The listing builds one solid part. Answer for the finished solid, in the listing's coordinates (mm). A direction names the side the tool comes from. Round coordinates to 2 decimals unless told otherwise and drop trailing zeros. Write each loop counter-clockwise with the first axis right and the second up, starting at its lowest first coordinate (ties: lowest second). Pieces come first, ordered by that corner, then holes.
Item 1: Find section C-C on z = 15. Give the vertices of the cut face in (x, y) (1 decimal).
Item 2: Find section B-B on y = 9. Give the vertices of the cut face in (x, z), then the cut area to 3 significant figures.
Item 3: A tool of negligible diameter and unlimited length cuts with its end or side. For faces 1 (the face through (13.694, 27.716, 14.79)), 2 (the face through (8.58, 15.86, 14.79)), 3 (the face through (14.315, 18.679, 14.79)), from which of +Z, -Z, +X, -X, +Y, -Y can it reach the whole face along a straight path? Write none if from no direction.
Item 4: Each of these flat-tipped pins is pushed along its axis until it touches: pin 1 (5 mm diameter, centred on y = 19, z = 20.5, fed in from -X); pin 2 (8 mm diameter, centred on x = 22.5, z = 10, fed in from +Y); pin 3 (5 mm diameter, centred on y = 25.5, z = 26.5, fed in from +X). Where does it stop, or does it pass through?
Item 5: For a pull along Y with two mould halves and no side action, classify faces 4 (the face through (17, 0, 15)), 5 (the face through (7.846, 28.994, 14.79)), 6 (the face through (4.78, 3.05, 14.79)) as +Y half, -Y half, draft (parallel to the pull), parting line (faces both ways), or undercut.
Item 6: Find section A-A on x = 7.5. Give the vertices of the cut face in (y, z).
Item 7: Find the intervals of material crossed by probe 1 along Y at (x, z) = (27.25, 19.5); probe 2 along X at (y, z) = (4.25, 15); probe 3 along X at (y, z) = (16.5, 23.25), in increasing order.
Item 8: Find section D-D on z = 26.5. Give the vertices of the cut face in (x, y) (1 decimal), then the cut area to 3 significant figures.
Autodesk Inventor part; units mm, degrees
ref_plane "YZ Plane" through (0, 0, 0) normal (1, 0, 0) x (0, 1, 0)
ref_plane "XZ Plane" through (0, 0, 0) normal (0, 1, 0) x (-1, 0, 0)
ref_plane "XY Plane" through (0, 0, 0) normal (0, 0, 1) x (1, 0, 0)
sketch "Szkic1" plane through (0, 0, 0) normal (0, 0, 1) x (1, 0, 0)
  line L0 (0, -6.7527) -> (0, 35.3194)
  line L1 (0.8414, 3.8525) -> (6.4011, 29.3091)
  line L2 (6.4011, 29.3091) -> (9.3321, 28.669)
  line L3 (9.3321, 28.669) -> (3.9978, 4.2447)
  line L4 (5.9517, 3.818) -> (11.286, 28.2423)
  line L5 (11.286, 28.2423) -> (16.1709, 27.1754)
  arc A0 (3.9978, 4.2447) -> (5.9517, 3.818) centre (4.9747, 4.0314) ccw
  line L6 (16.1709, 27.1754) -> (12.4071, 9.942)
  line L7 (13.9707, 8) -> (30.48, 8)
  arc A1 (12.4071, 9.942) -> (13.9707, 8) centre (13.9707, 9.6005) ccw
  line L8 (3.9433, 0) -> (30.48, 0)
  line L9 (30.48, 0) -> (30.48, 8)
  arc A2 (0.8414, 3.8525) -> (3.9433, 0) centre (3.9433, 3.175) ccw
  point P0 (0, 0)
  dimension "d0" = 12.32
  dimension "d1" = 3
  dimension "d2" = 30
  dimension "d3" = 5
  dimension "d4" = 8
  dimension "d5" = 25
  dimension "d6" = 2
  dimension "d7" = 30.48
  dimension "d8" = 1.6005
  dimension "d9" = 3.175
extrude "Wyciągnięcie proste1" add sketch "Szkic1" along normal blind 30
sketch "Szkic2" plane through (13.9707, 8, 0) normal (0, 1, 0) x (1, 0, 0)
  circle A0 centre (8.4108, -15) radius 2.25
  point P0 (-13.9707, 0)
  dimension "d12" = 4.5
extrude "Wyciągnięcie proste2" cut sketch "Szkic2" against normal blind 30
sketch "Szkic3" plane through (16.1709, 27.1754, 30) normal (0.9769712, -0.2133714, 0) x (0, 0, -1)
  circle A0 centre (15, -6.4184) radius 1.45
  point P0 (30, -30)
  dimension "d15" = 2.9
extrude "Wyciągnięcie proste3" cut sketch "Szkic3" against normal up to next
properties part number "lustereczko"
Check values:
1. outline: (0.8, 3.9) arc R3.2 ccw to (3.9, 0) - (20.1, 0) - (20.1, 8) - (14, 8) arc R1.6 cw to (12.4, 9.9) - (14.5, 19.5) - (9.6, 20.6) - (6, 3.8) arc R1 cw to (4, 4.2) - (9.3, 28.7) - (6.4, 29.3) - close; (10.2, 23.4) - (15.1, 22.3) - (16.2, 27.2) - (11.3, 28.2) - close; (24.6, 0) - (30.5, 0) - (30.5, 8) - (24.6, 8) - close
2. outline: (1.97, 0) - (5.04, 0) - (5.04, 30) - (1.97, 30) - close; (7.08, 0) - (12.49, 0) - (12.49, 30) - (7.08, 30) - close
2. area: 254 mm2
3. face 1: +Z, -Z, +X, +Y
3. face 2: +Z, -Z
3. face 3: +Z, -Z, +X
4. pin 1: stops at x = 3.6
4. pin 2: stops at y = 8
4. pin 3: stops at x = 16.17
5. face 4: -Y half
5. face 5: +Y half
5. face 6: undercut
6. outline: (0, 0) - (10.91, 0) - (10.91, 30) - (0, 30) - close; (20.28, 0) - (29.07, 0) - (29.07, 30) - (20.28, 30) - close
7. probe 1: y = 0 to 8
7. probe 2: x = 0.93 to 4, 6.05 to 20.13, 24.63 to 30.48
7. probe 3: x = 3.6 to 6.67, 8.72 to 13.84
8. outline: (0.8, 3.9) arc R3.2 ccw to (3.9, 0) - (30.5, 0) - (30.5, 8) - (14, 8) arc R1.6 cw to (12.4, 9.9) - (16.2, 27.2) - (11.3, 28.2) - (6, 3.8) arc R1 cw to (4, 4.2) - (9.3, 28.7) - (6.4, 29.3) - close
8. area: 390 mm2
